```python
from build123d import *

# Parameters (mm, degrees)
SKETCH1_W           = 25.4
SKETCH1_H           = 25.4
SKETCH1_W_2         = 20.32
SKETCH1_H_2         = 20.32
BOSS_EXTRUDE2_DEPTH = 74.168
FILLET1_R           = 1.27


with BuildPart() as part:
    # Sketch1 → Boss-Extrude2 (new body)
    with BuildSketch(Plane.XY.offset(-3.048)):
        Rectangle(SKETCH1_W, SKETCH1_H)
        Rectangle(SKETCH1_W_2, SKETCH1_H_2, mode=Mode.SUBTRACT)
    extrude(amount=BOSS_EXTRUDE2_DEPTH)

    # Fillet1
    fillet1_edges = [part.edges().sort_by_distance(p)[0] for p in [
        (-12.7, 12.7, 34.036),
        (-12.7, -12.7, 34.036),
        (12.7, -12.7, 34.036),
        (12.7, 12.7, 34.036),
        (-10.16, -10.16, 34.036),
        (10.16, -10.16, 34.036),
        (10.16, 10.16, 34.036),
        (-10.16, 10.16, 34.036),
    ]]
    fillet(fillet1_edges, radius=FILLET1_R)


solid = part.part
```
CAD build for the part. Positions are in the model's coordinates, mm. A direction names the side the tool comes from. Round coordinates to 2 decimals unless told otherwise and drop trailing zeros. Loops run counter-clockwise (first coordinate to the right, second up) from the corner with the lowest first, then second, coordinate; pieces in that order, holes last. Notation, with made-up numbers: M -34,9.25 L 16,9.25 A31 ccw 16,43.25 Z; hole C 79,1 d11. An arc over 180 degrees is marked long. Use a Markdown table: item, result. Add a question column.
(1) Cut at C-C (z = 17.5). Give the cut face in (x, y).
(2) Pull direction Y, two halves, no side cores. Call faces 3 (the face through (-9.778, 9.798, 34.555)), 4 (the face through (0, 10.16, 34)), 5 (the face through (-12.7, 0, 34)), 6 (the face through (-12.338, -12.318, 34.555)): +Y half, -Y half, draft (parallel to the pull), parting line (faces both ways), or undercut.
(3) Flat gauge pin, fed straight in: pin 1 (1 mm diameter, centred on x = 8, y = 4, fed in from +Z). Where does the tip first touch, or does it go through?
(4) Which spindle directions (+Z, -Z, +X, -X, +Y, -Y) get a long thin tool onto all of the face, cutting with end or side? Do faces 1 (the face through (-10.16, 0, 34)), 2 (the face through (12.318, 12.338, 34.555)). Say none if no direction does.
(5) Cut at A-A (x = -7.5). Give the cut face in (y, z).
(6) Drill centre lines: line 1 (Y direction, x = 4.5, z = 56); line 2 (X direction, y = 11.5, z = 31.5). Where is each one in solid material? Low to high.
Geometry says:
| question | item | result |
|---|---|---|
| 1 | outline | M -12.7,-11.43 A1.27 ccw -11.43,-12.7 L 11.43,-12.7 A1.27 ccw 12.7,-11.43 L 12.7,11.43 A1.27 ccw 11.43,12.7 L -11.43,12.7 A1.27 ccw -12.7,11.43 Z; hole M -10.16,-8.89 A1.27 ccw -8.89,-10.16 L 8.89,-10.16 A1.27 ccw 10.16,-8.89 L 10.16,8.89 A1.27 ccw 8.89,10.16 L -8.89,10.16 A1.27 ccw -10.16,8.89 Z |
| 2 | face 3 | undercut |
| 2 | face 4 | undercut |
| 2 | face 5 | draft |
| 2 | face 6 | -Y half |
| 3 | pin 1 | passes through |
| 4 | face 1 | +Z, -Z |
| 4 | face 2 | +Z, -Z, +X, +Y |
| 5 | outline | M -12.7,-3.05 L -10.16,-3.05 L -10.16,71.12 L -12.7,71.12 Z; M 10.16,-3.05 L 12.7,-3.05 L 12.7,71.12 L 10.16,71.12 Z |
| 6 | line 1 | y = -12.7 to -10.16, 10.16 to 12.7 |
| 6 | line 2 | x = -12.7 to 12.7 |
